Design review of the part built by this model. Coordinates are the model's own, in mm. A direction names the side the tool comes from. Coordinates: 2 decimals unless noted, no trailing zeros. Loops run counter-clockwise (first coordinate to the right, second up) from the corner with the lowest first, then second, coordinate; pieces in that order, holes last.
from build123d import *

# Parameters (mm, degrees)
SALIENTE_EXTRUIR1_DEPTH                        = 8
CROQUIS2_R                                     = 1.75
SALIENTE_EXTRUIR2_DEPTH                        = 2
PERFORADOR_PARA_ROSCAR_PARA_MACHO_DE_ROS_D     = 3.3
PERFORADOR_PARA_ROSCAR_PARA_MACHO_DE_ROS_DEPTH = 7
PERFORADOR_PARA_ROSCAR_PARA_MACHO_DE_ROS_TIP   = 0.991420021


with BuildPart() as part:
    # Croquis1 → Saliente-Extruir1 (new body)
    with BuildSketch(Plane.XY):
        with BuildLine():
            Line((-21.62608642, 28.286151185), (-8.859820947, 2.289392402))
            ThreePointArc((-8.859820947, 2.289392402), (-10.687098367, -3.064209864), (-16.040700634, -1.236932444))
            Line((-16.040700634, -1.236932444), (-28.162442293, 23.44734148))
            add(Edge.make_bspline(
                [(-28.162442293, 23.44734148), (-41.803068248, 51.224616152), (-38.554014675, 17.849905123)],
                knots=[2.065965679, 2.065965679, 2.065965679, 4.571411553, 4.571411553, 4.571411553], degree=2, weights=[1, 0.312737171, 1]))
            Line((-38.554014675, 17.849905123), (-38.554014675, -9.292104706))
            Line((-38.554014675, -9.292104706), (-43.554014675, -10.899488854))
            Line((-43.554014675, -10.899488854), (-43.554014675, 23.192572958))
            ThreePointArc((-43.554014675, 23.192572958), (-34.613059385, 34.4484445), (-21.62608642, 28.286151185))
        make_face()
    extrude(amount=SALIENTE_EXTRUIR1_DEPTH)

    # Croquis2 → Saliente-Extruir2 (add)
    with BuildSketch(Plane.XY.offset(8)):
        with Locations((-12.45026079, 0.526229979)):
            Circle(CROQUIS2_R)
    saliente_extruir2 = extrude(amount=SALIENTE_EXTRUIR2_DEPTH)

    # Simetría1: Saliente-Extruir2 across plane
    add(saliente_extruir2.mirror(Plane.XY.offset(4)))

    # Perforador para roscar para macho de roscar para M41
    with Locations(Plane.ZY.offset(43.554014675)):
        with Locations((4, -6.399488854)):
            Hole(PERFORADOR_PARA_ROSCAR_PARA_MACHO_DE_ROS_D / 2, depth=PERFORADOR_PARA_ROSCAR_PARA_MACHO_DE_ROS_DEPTH)
            with Locations((0, 0, -(PERFORADOR_PARA_ROSCAR_PARA_MACHO_DE_ROS_DEPTH + PERFORADOR_PARA_ROSCAR_PARA_MACHO_DE_ROS_TIP / 2))):  # 118° drill point
                Cone(0, PERFORADOR_PARA_ROSCAR_PARA_MACHO_DE_ROS_D / 2, PERFORADOR_PARA_ROSCAR_PARA_MACHO_DE_ROS_TIP, mode=Mode.SUBTRACT)


solid = part.part
Q1. Machinability: for faces 5 (the flat face through (-22, 10.9, 3.9)), 6 (the cylindrical face through (-14.2, 0.6, 9)), 7 (the cylindrical face through (-41.019, -5.284, 5.216)), which of the approach directions +Z, -Z, +X, -X, +Y, -Y give a long, thin tool a straight path to every point of the face, cutting with its end or side? Answer none if there is none.
Q2. Take a section at A-A, the plane y = 3. Write out the cut boundary in (x, z).
Q3. For line 1 (Y direction, x = -42.4, z = 4); line 2 (X direction, y = 11.5, z = 0.5); line 3 (Z direction, x = -41, y = 22.5), list the stretches that pass through material, from the lowest coordinate up.
Q4. Take a section at C-C, the plane z = -1. Write out the cut boundary in (x, y).
Q5. Take a section at B-B, the plane x = -12. Write out the cut boundary in (y, z).
Q6. The part is to be moulded in two halves that separate along X. For faces 1 (the cylindrical face through (-10.609, -3.025, 3.944)), 2 (the flat face through (-12, 1, -2)), 3 (the flat face through (-38.554, 4, 4)), 4 (the cylindrical face through (-14.2, 0.6, -1)), say which applies: pulls with the +X half, pulls with the -X half, needs draft (parallel to the pull), parting line crosses it, or undercut.
Q7. Take a section at D-D, the plane x = -23. Write out the cut boundary in (y, z), then the cut area to 3 significant figures.
Q8. Clearance check with flat-ended pins moving along their axes: pin 1 Ø17.5 at (x, y) = (-22.5, 21) entering from -Z; pin 2 Ø2 at (x, z) = (-21.5, 1) entering from +Y; pin 3 Ø4 at (y, z) = (3.5, 3.5) entering from +X; pin 4 Ø3 at (x, y) = (-36.5, 12) entering from -Z. State where each tip first meets the part, or that it passes through.
Entries:
1. face 5: +Z, -Z, -Y
1. face 6: +Z
1. face 7: +X, -X
2. outline: (-43.55, 0) - (-38.55, 0) - (-38.55, 8) - (-43.55, 8) - close; (-18.12, 0) - (-9.21, 0) - (-9.21, 8) - (-18.12, 8) - close
3. line 1: y = -10.53 to -8.05, -4.75 to 28.23
3. line 2: x = -43.55 to -38.55, -22.3 to -13.38
3. line 3: z = 0 to 8
4. outline: circle Ø3.5 at (-12.45, 0.53)
5. outline: (-3.45, 0) - (-1.16, 0) - (-1.16, -2) - (2.22, -2) - (2.22, 0) - (8.68, 0) - (8.68, 8) - (2.22, 8) - (2.22, 10) - (-1.16, 10) - (-1.16, 8) - (-3.45, 8) - close
6. face 1: undercut
6. face 2: needs draft
6. face 3: undercut
6. face 4: parting line crosses it
7. outline: (12.93, 0) - (30.44, 0) - (30.44, 8) - (12.93, 8) - close
7. area: 140 mm2
8. pin 1: stops at z = 0
8. pin 2: stops at y = 29.77
8. pin 3: stops at x = -8.57
8. pin 4: passes through
